```python
from build123d import *

# Parameters (mm, degrees)
SKETCH2_R          = 3.5
CUT_EXTRUDE1_DEPTH = 20


with BuildPart() as part:
    # Sketch1 → Revolve1 (revolve)
    with BuildSketch(Plane.XY):
        with BuildLine():
            Line((12.5, -14.9725871), (17.43319678, -14.9725871))
            Line((17.43319678, -14.9725871), (47.5, -14.9725871))
            Line((47.5, -14.9725871), (47.5, 0.0274129))
            Line((47.5, 0.0274129), (23.392075087, 0.0274129))
            Line((23.392075087, 0.0274129), (23.392075087, 88.874931748))
            ThreePointArc((23.392075087, 88.874931748), (23.040193106, 89.436291225), (22.381592941, 89.364241145))
            ThreePointArc((22.381592941, 89.364241145), (15.113172999, 80.869909317), (12.5, 70))
            Line((12.5, 70), (12.5, 0))
            Line((12.5, 0), (0, 0))
            Line((0, 0), (0, -14.9725871))
            Line((0, -14.9725871), (12.5, -14.9725871))
        make_face()
    revolve(axis=Axis((0, 0, 0), (0, -1, 0)))

    # Sketch2 → Cut-Extrude1 (cut)
    with BuildSketch(Plane(origin=(0, 0.0274129, 0), x_dir=(1, 0, 0), z_dir=(0, 1, 0))):
        with Locations((-2.39741815, 35.920083327)):
            Circle(SKETCH2_R)
        with Locations((-35.920083327, -2.39741815)):
            Circle(SKETCH2_R)
        with Locations((2.39741815, -35.920083327)):
            Circle(SKETCH2_R)
        with Locations((35.920083327, 2.39741815)):
            Circle(SKETCH2_R)
    extrude(amount=-CUT_EXTRUDE1_DEPTH, mode=Mode.SUBTRACT)


solid = part.part
```
Model file for the job. Use its own axes, mm. A direction names the side the tool comes from. Give positions to 0.01 mm unless a question says otherwise; leave off trailing zeros. Loops run counter-clockwise (first coordinate to the right, second up) from the corner with the lowest first, then second, coordinate; pieces in that order, holes last. Notation, with made-up numbers: (14, 50) - (43, 50) arc R12 ccw to (43, 66) - close; hole circle Ø4 at (11.5, 32). An arc over 180 degrees is marked (long way). One line per item, written item: value. Start each with the question number.
1. Slice it at A-A (y = 59.5). List the corners of the cut face in (x, z).
2. Slice it at C-C (y = 82). List the corners of the cut face in (x, z).
3. Probe L1, parallel to Z at x = 0, y = 25; L2, parallel to Y at x = -22, z = -27; L3, parallel to Z at x = 2, y = 52.5. List the from-to ranges inside material, lowest first. Write a range as from..to.
4. Pin check, flat tips, straight feed: pin 1 (8 mm diameter, centred on y = 45.5, z = 7, fed in from +X); pin 2 (2 mm diameter, centred on x = -6, y = 10, fed in from +Z); pin 3 (4 mm diameter, centred on y = 78.5, z = -16, fed in from -X). Stop position of each tip, or through.
5. Which spindle directions (+Z, -Z, +X, -X, +Y, -Y) get a long thin tool onto all of the face, cutting with end or side? Do faces 4 (the cylindrical face through (-17.24, 45.07, 15.81)), 5 (the cylindrical face through (-39.417, -7.368, 2.244)). Say none if no direction does.
6. Slice it at B-B (x = 28). List the corners of the cut face in (y, z).
7. Pull direction X, two halves, no side cores. Call faces 1 (the flat face through (10, 0.027, 22)), 2 (the cylindrical face through (32.423, -7.368, -2.551)), 3 (the cylindrical face through (-10.3, -7.37, -46.37)): pulls with the +X half, pulls with the -X half, needs draft (parallel to the pull), parting line crosses it, or undercut.
Solution:
1. outline: circle Ø46.78 at (0, 0); hole circle Ø25 at (0, 0)
2. outline: circle Ø46.78 at (0, 0); hole circle Ø31.46 at (0, 0)
3. L1: z = -23.39..-12.5, 12.5..23.39
3. L2: y = -14.97..0.03
3. L3: z = -23.31..-12.34, 12.34..23.31
4. pin 1: stops at x = 23.2
4. pin 2: stops at z = 22.85
4. pin 3: stops at x = -18.74
5. face 4: +Y
5. face 5: +Y, -Y
6. outline: (-14.97, -38.37) - (0.03, -38.37) - (0.03, 38.37) - (-14.97, 38.37) - close
7. face 1: needs draft
7. face 2: undercut
7. face 3: parting line crosses it
